Here's the drawing with two shaded views (mm, measured from the low corner). I have some questions. A direction names the side the tool comes from. Round coordinates to 2 decimals unless told otherwise and drop trailing zeros. Loops run counter-clockwise (first coordinate to the right, second up) from the corner with the lowest first, then second, coordinate; pieces in that order, holes last.
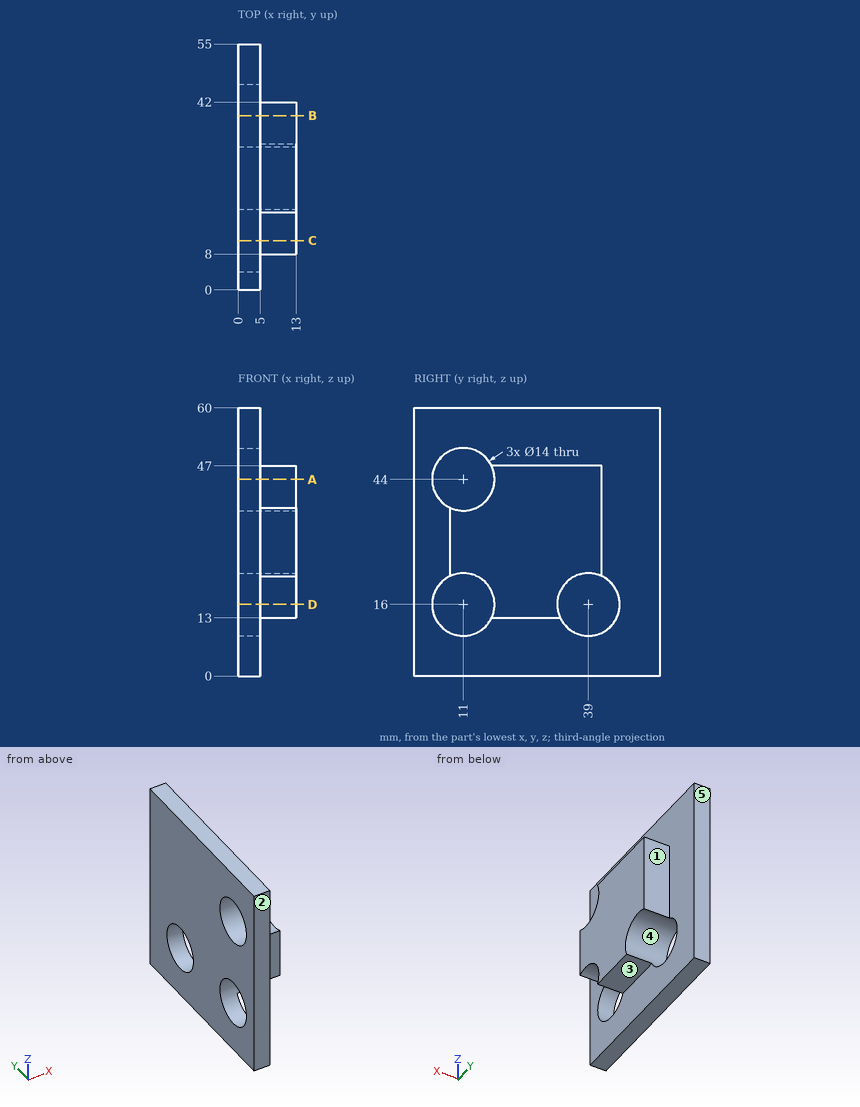
Item 1: If I drill on line 1 along Y through (x, z) = (2.75, 16); line 2 along Z through (x, y) = (4.5, 11); line 3 along Z through (x, y) = (3.75, 15.5), over which ranges is the centre line in solid material (lowest first)?
Results list:
line 1: y = 0 to 4, 18 to 32, 46 to 55
line 2: z = 0 to 9, 23 to 37, 51 to 60
line 3: z = 0 to 10.64, 21.36 to 38.64, 49.36 to 60
Item 2: If we section it at A-A, the plane z = 44: Please give me the cut outline in (x, y).
Results list:
outline: (0, 0) - (5, 0) - (5, 4) - (0, 4) - close; (0, 18) - (13, 18) - (13, 42) - (5, 42) - (5, 55) - (0, 55) - close
Item 3: For the marked faces 1 and 2, which set-ups out of +Z, -Z, +X, -X, +Y, -Y let a thin tool reach every point of the face, with its end or its side?
Results list:
face 1: +Z, -Z, +X, +Y
face 2: +Z, -Z, +X, -X, -Y
Item 4: We'd pull the mould along Y, two halves only. Please class the marked faces 3, 4 and 5: released by +Y, released by -Y, zero draft, split by the parting line, or undercut.
Results list:
face 3: zero draft
face 4: undercut
face 5: released by +Y
Item 5: If we section it at C-C, the plane y = 11: Please give me the cut outline in (x, z), then the cut area to 3 significant figures.
Results list:
outline: (0, 0) - (5, 0) - (5, 9) - (0, 9) - close; (0, 23) - (13, 23) - (13, 37) - (0, 37) - close; (0, 51) - (5, 51) - (5, 60) - (0, 60) - close
area: 272 mm2
Item 6: If we section it at D-D, the plane z = 16: Please give me the cut outline in (x, y).
Results list:
outline: (0, 0) - (5, 0) - (5, 4) - (0, 4) - close; (0, 18) - (13, 18) - (13, 32) - (0, 32) - close; (0, 46) - (5, 46) - (5, 55) - (0, 55) - close
Item 7: Will these pins go through, and if not, where does the flat tip stop? pin 1 (2.5 mm diameter, centred on x = 10.5, y = 23, fed in from -Z); pin 2 (6.5 mm diameter, centred on x = 10.5, y = 32.5, fed in from +Z); pin 3 (12 mm diameter, centred on y = 46.5, z = 13.5, fed in from +X).
Results list:
pin 1: stops at z = 13
pin 2: stops at z = 47
pin 3: stops at x = 5
Item 8: If we section it at B-B, the plane y = 39: Please give me the cut outline in (x, z), then the cut area to 3 significant figures.
Results list:
outline: (0, 0) - (5, 0) - (5, 9) - (0, 9) - close; (0, 23) - (13, 23) - (13, 47) - (5, 47) - (5, 60) - (0, 60) - close
area: 422 mm2
